Input: part model. Units: mm. Frame: model coordinates. A direction names the side the tool comes from. Coordinates: 2 decimals unless noted, no trailing zeros. Order: outer loops, then holes, each group sorted by start corner. A loop starts at its lowest first (then second) coordinate and runs counter-clockwise, first axis right, second up. Notation, with made-up numbers: (-4, -34.75) - (9, -34.75) arc R24 ccw to (9, -17.75) - close; hole circle Ø2 at (17.5, 67.5). An arc over 180 degrees is marked (long way). One line per question, with ' | ' between items.
from build123d import *

# Parameters (mm, degrees)
SKETCH1_W                 = 711.2
SKETCH1_H                 = 50.8
BOSS_EXTRUDE1_DEPTH       = 25.4
SKETCH2_W                 = 20.32
SKETCH2_H                 = 45.72
CUT_EXTRUDE1_DEPTH        = 712.2
F_6_CLEARANCE_HOLE1_D     = 4.1402
F_6_CLEARANCE_HOLE1_DEPTH = 50.8
F_6_CLEARANCE_HOLE2_D     = 4.1402
F_6_CLEARANCE_HOLE2_DEPTH = 50.8
FILLET1_R                 = 0.5
FILLET2_R                 = 2.54


with BuildPart() as part:
    # Sketch1 → Boss-Extrude1 (new body)
    with BuildSketch(Plane(origin=(12.7, 0, 0), x_dir=(0, 0, -1), z_dir=(1, 0, 0))):
        Rectangle(SKETCH1_W, SKETCH1_H)
    extrude(amount=-BOSS_EXTRUDE1_DEPTH)

    # Sketch2 → Cut-Extrude1 (cut, through all)
    with BuildSketch(Plane(origin=(0, 0, -355.6), x_dir=(-1, 0, 0), z_dir=(0, 0, -1))):
        Rectangle(SKETCH2_W, SKETCH2_H)
    extrude(amount=-CUT_EXTRUDE1_DEPTH, mode=Mode.SUBTRACT)

    # #6 Clearance Hole1
    with Locations(Plane(origin=(0, -25.4, 0), x_dir=(-1, 0, 0), z_dir=(0, -1, 0))):
        with Locations((0, 711.2), (0, 736.6), (0, 685.8), (0, 660.4), (0, 635), (0, 609.6), (0, 584.2), (0, 558.8), (0, 533.4), (0, 508), (0, 482.6), (0, 457.2), (0, 431.8), (0, 406.4), (0, 381), (0, 355.6), (0, 330.2), (0, 304.8), (0, 279.4), (0, 254), (0, 228.6), (0, 203.2), (0, 177.8), (0, 152.4), (0, 127), (0, 101.6), (0, 76.2), (0, 50.8), (0, 25.4), (0, 0), (0, -25.4), (0, -50.8), (0, -76.2), (0, -101.6), (0, -127), (0, -152.4), (0, -177.8), (0, -203.2), (0, -228.6), (0, -254), (0, -279.4), (0, -304.8), (0, -330.2), (0, -355.6), (0, -381), (0, -406.4), (0, -431.8), (0, -457.2), (0, -482.6), (0, -508), (0, -533.4), (0, -558.8), (0, -584.2), (0, -609.6), (0, -635), (0, -660.4), (0, -685.8), (0, -711.2), (0, -736.6)):
            Hole(F_6_CLEARANCE_HOLE1_D / 2, depth=F_6_CLEARANCE_HOLE1_DEPTH)

    # #6 Clearance Hole2
    with Locations(Plane(origin=(0, 25.4, 0), x_dir=(1, 0, 0), z_dir=(0, 1, 0))):
        with Locations((0, 711.2), (0, 736.6), (0, 685.8), (0, 660.4), (0, 635), (0, 609.6), (0, 584.2), (0, 558.8), (0, 533.4), (0, 508), (0, 482.6), (0, 457.2), (0, 431.8), (0, 406.4), (0, 381), (0, 355.6), (0, 330.2), (0, 304.8), (0, 279.4), (0, 254), (0, 228.6), (0, 203.2), (0, 177.8), (0, 152.4), (0, 127), (0, 101.6), (0, 76.2), (0, 50.8), (0, 25.4), (0, 0), (0, -25.4), (0, -50.8), (0, -76.2), (0, -101.6), (0, -127), (0, -152.4), (0, -177.8), (0, -203.2), (0, -228.6), (0, -254), (0, -279.4), (0, -304.8), (0, -330.2), (0, -355.6), (0, -381), (0, -406.4), (0, -431.8), (0, -457.2), (0, -482.6), (0, -508), (0, -533.4), (0, -558.8), (0, -584.2), (0, -609.6), (0, -635), (0, -660.4), (0, -685.8), (0, -711.2), (0, -736.6)):
            Hole(F_6_CLEARANCE_HOLE2_D / 2, depth=F_6_CLEARANCE_HOLE2_DEPTH)

    # Fillet1
    fillet1_edges = [part.edges().sort_by_distance(p)[0] for p in [
        (-10.16, -22.86, 0),
        (10.16, -22.86, 0),
        (10.16, 22.86, 0),
        (-10.16, 22.86, 0),
    ]]
    fillet(fillet1_edges, radius=FILLET1_R)

    # Fillet2
    fillet2_edges = [part.edges().sort_by_distance(p)[0] for p in [
        (-12.7, 25.4, 0),
        (-12.7, -25.4, 0),
        (12.7, 25.4, 0),
        (12.7, -25.4, 0),
    ]]
    fillet(fillet2_edges, radius=FILLET2_R)


solid = part.part
Item 1: Section B-B on z = -191.5. Return the cut outline in (x, y).
Data:
outline: (-12.7, -22.86) arc R2.54 ccw to (-10.16, -25.4) - (10.16, -25.4) arc R2.54 ccw to (12.7, -22.86) - (12.7, 22.86) arc R2.54 ccw to (10.16, 25.4) - (-10.16, 25.4) arc R2.54 ccw to (-12.7, 22.86) - close; hole (-10.16, -22.36) arc R0.5 ccw to (-9.66, -22.86) - (9.66, -22.86) arc R0.5 ccw to (10.16, -22.36) - (10.16, 22.36) arc R0.5 ccw to (9.66, 22.86) - (-9.66, 22.86) arc R0.5 ccw to (-10.16, 22.36) - close
Item 2: Section A-A on y = 10. Return the cut outline in (x, z).
Data:
outline: (-12.7, -355.6) - (-10.16, -355.6) - (-10.16, 355.6) - (-12.7, 355.6) - close; (10.16, -355.6) - (12.7, -355.6) - (12.7, 355.6) - (10.16, 355.6) - close
Item 3: Ray query, line 1 (X direction, y = -0.5, z = -158); line 2 (Y direction, x = -0.25, z = 95.5); line 3 (X direction, y = 23.55, z = 152.4). Return the intervals inside material, ascending.
Data:
line 1: -12.7 to -10.16, 10.16 to 12.7 | line 2: -25.4 to -22.86, 22.86 to 25.4 | line 3: -12.6 to -2.07, 2.07 to 12.6
Item 4: Contact query for a flat-ended pin moving along its axis: P1, Ø2.5, axis at x = 0, z = 330.2, coming from the -Y side. Output: stop coordinate, or through.
Data:
P1: through
Item 5: Draft query along X for faces 1 (the face through (12.7, 0, 5)), 2 (the face through (0, -25.4, 5)), 3 (the face through (0, -22.86, -5)), 4 (the face through (-12.7, 0, 5)). Return one class per face: released by +X, released by -X, zero draft, split by the parting line, or undercut.
Data:
face 1: released by +X | face 2: zero draft | face 3: undercut | face 4: released by -X
Item 6: Access query for faces 5 (the face through (10.16, 0, -5)), 6 (the face through (0, 25.4, 5)). Directions: +Z, -Z, +X, -X, +Y, -Y. A direction counts if a zero-diameter tool reaches every point of the face in a straight line with its end or side. Return the directions, or none.
Data:
face 5: +Z, -Z | face 6: +Z, -Z, +X, -X, +Y
